Can you work these out from the model? Positions are in its coordinate system, mm. A direction names the side the tool comes from. Round coordinates to 2 decimals unless told otherwise and drop trailing zeros. Write each loop counter-clockwise with the first axis right and the second up, starting at its lowest first coordinate (ties: lowest second). Pieces come first, ordered by that corner, then holes. Notation, with made-up numbers: M -11,-5.75 L 10,-5.75 A28 ccw 10,23.25 Z; hole C -28,30 d4. An arc over 180 degrees is marked long. Answer in a Markdown table with one row per item. Add a question column.
(1) Suppose I cut it at C-C, the plane y = 21. Write out the boundary of the cut face in (x, z) (3 decimals).
(2) If I drill on probe 1 along X at (y, z) = (21, 4.5) (3 decimals); probe 2 along Y at (x, z) = (11.25, 5.5); probe 3 along X at (y, z) = (2.5, 0.5), over which ranges is the centre line in solid material (lowest first)?
(3) For faces 4 (the face through (24.892, 24, 3)), 5 (the face through (12, 46.66, 3)), which set-ups out of +Z, -Z, +X, -X, +Y, -Y let a thin tool reach every point of the face, with its end or its side?
(4) Suppose I cut it at A-A, the plane x = 12.75. Write out the boundary of the cut face in (y, z), then the cut area to 3 significant figures.
(5) Suppose I cut it at B-B, the plane z = 3. Write out the boundary of the cut face in (x, y) (3 decimals).
(6) If we mould it in two halves opening along X, with no side actions, what happens to faces 1 (the face through (17.46, 45.754, 3.131)), 2 (the face through (12, 48.692, 3)), 3 (the face through (0, 24, 3))? For each: released by +X, released by -X, zero draft, split by the parting line, or undercut.
from build123d import *

# Parameters (mm, degrees)
F0_W     = 24.892
F0_H     = 48.6918
F1_DEPTH = 6.35


with BuildPart() as f1:
    # F0 (on Top) → F1 (new body)
    with BuildSketch(Plane.XY):
        with Locations((12.446, 24.3459)):
            Rectangle(F0_W, F0_H)
        with BuildLine():
            ThreePointArc((6.477, 43.4848), (7.406936, 45.729864), (9.652, 46.6598))
            Line((9.652, 46.6598), (15.24, 46.6598))
            ThreePointArc((15.24, 46.6598), (17.485064, 45.729864), (18.415, 43.4848))
            Line((18.415, 43.4848), (18.415, 5.207))
            ThreePointArc((18.415, 5.207), (17.485064, 2.961936), (15.24, 2.032))
            Line((15.24, 2.032), (9.652, 2.032))
            ThreePointArc((9.652, 2.032), (7.406936, 2.961936), (6.477, 5.207))
            Line((6.477, 5.207), (6.477, 43.4848))
        make_face(mode=Mode.SUBTRACT)
    extrude(amount=F1_DEPTH)


solid = f1.part
Calculated:
| question | item | result |
|---|---|---|
| 1 | outline | M 0,0 L 6.477,0 L 6.477,6.35 L 0,6.35 Z; M 18.415,0 L 24.892,0 L 24.892,6.35 L 18.415,6.35 Z |
| 2 | probe 1 | 0 to 6.477, 18.415 to 24.892 |
| 2 | probe 2 | 0 to 2.03, 46.66 to 48.69 |
| 2 | probe 3 | 0 to 7.99, 16.9 to 24.89 |
| 3 | face 4 | +Z, -Z, +X, +Y, -Y |
| 3 | face 5 | +Z, -Z |
| 4 | outline | M 0,0 L 2.03,0 L 2.03,6.35 L 0,6.35 Z; M 46.66,0 L 48.69,0 L 48.69,6.35 L 46.66,6.35 Z |
| 4 | area | 25.8 mm² |
| 5 | outline | M 0,0 L 24.892,0 L 24.892,48.692 L 0,48.692 Z; hole M 6.477,5.207 A3.175 ccw 9.652,2.032 L 15.24,2.032 A3.175 ccw 18.415,5.207 L 18.415,43.485 A3.175 ccw 15.24,46.66 L 9.652,46.66 A3.175 ccw 6.477,43.485 Z |
| 6 | face 1 | undercut |
| 6 | face 2 | zero draft |
| 6 | face 3 | released by -X |
